Source: three-view drawing plus pictorial views. Frame: mm from the lowest corner of the part. Give positions to 0.01 mm unless a question says otherwise; leave off trailing zeros. Order: outer loops, then holes, each group sorted by start corner. A loop starts at its lowest first (then second) coordinate and runs counter-clockwise, first axis right, second up.
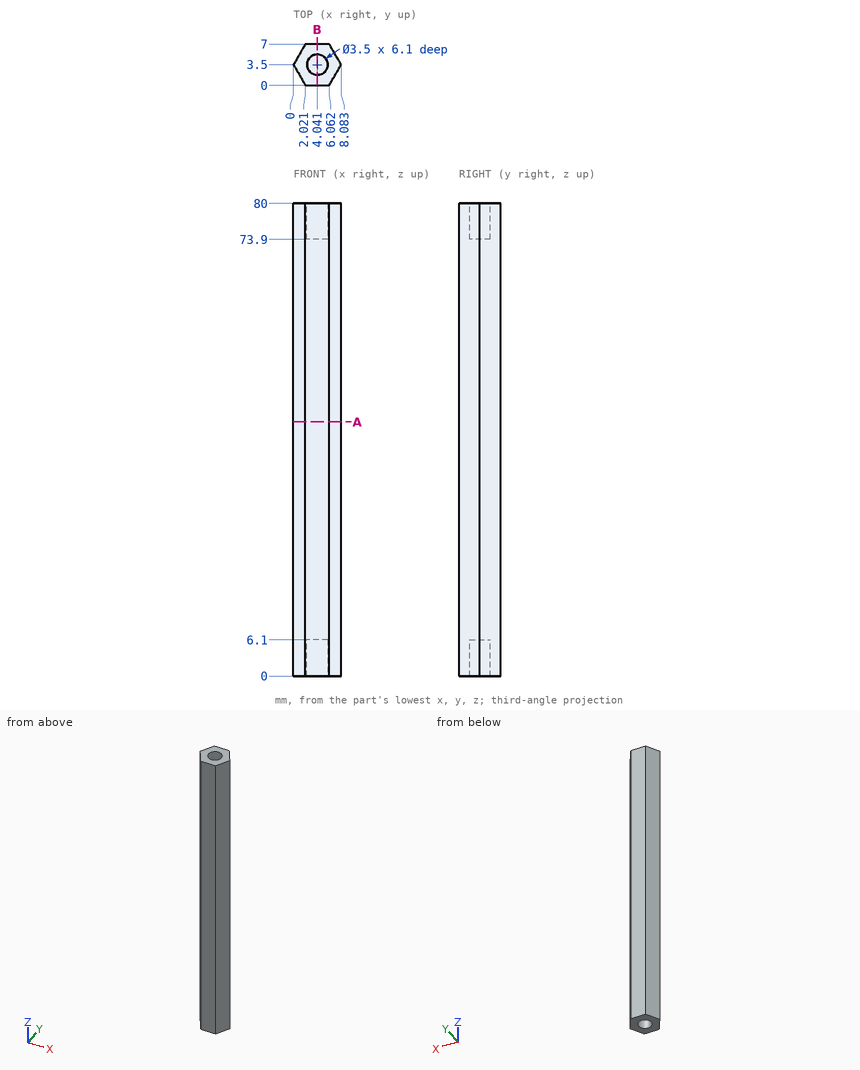
1) Section query A-A on z = 43. Output: boundary loops of the cut face in (x, y).
Checks:
outline: (0, 3.5) - (2.02, 0) - (6.06, 0) - (8.08, 3.5) - (6.06, 7) - (2.02, 7) - close
2) Section query B-B on x = 4. Output: boundary loops of the cut face in (y, z), and give its area (3 significant figures).
Checks:
outline: (0, 0) - (1.75, 0) - (1.75, 6.1) - (5.25, 6.1) - (5.25, 0) - (7, 0) - (7, 80) - (5.25, 80) - (5.25, 73.9) - (1.75, 73.9) - (1.75, 80) - (0, 80) - close
area: 517 mm2
3) First-contact query: pin 1 Ø1.5 at (y, z) = (5, 29.5) entering from -X; pin 2 Ø1.8 at (x, y) = (4.5, 3.5) entering from -Z. Flat tips, straight axial feed; report the tip coordinate or a pass-through.
Checks:
pin 1: stops at x = 0.43
pin 2: stops at z = 6.1
4) Ray query, L1, parallel to X at y = 3.5, z = 3; L2, parallel to Z at x = 5.5, y = 4; L3, parallel to X at y = 3.75, z = 72 (1 decimal). Return the intervals inside material, ascending.
Checks:
L1: x = 0 to 2.29, 5.79 to 8.08
L2: z = 6.1 to 73.9
L3: x = 0.1 to 7.9
